Part model, mm, in its own coordinate system. A direction names the side the tool comes from. Round coordinates to 2 decimals unless told otherwise and drop trailing zeros. Order: outer loops, then holes, each group sorted by start corner. A loop starts at its lowest first (then second) coordinate and runs counter-clockwise, first axis right, second up. Notation, with made-up numbers: (23, -5) - (28, -5) arc R16 cw to (28, 18) - close; hole circle Ø8 at (44.5, 41.25). An arc over 180 degrees is marked (long way). Answer as a JSON object with one key per item and string values.
```python
from build123d import *

# Parameters (mm, degrees)
F1_DEPTH = 5
F3_DEPTH = 100
F4_SIZE  = 1


with BuildPart() as f1:
    # F0 (on Front) → F1 (new body)
    with BuildSketch(Plane.XZ):
        Polygon((66.3298651576, -50.2631962299), (66.3298651576, 49.7368037701), (-33.6701348424, 49.7368037701), (-33.6701348424, -50.2631962299), (-3.6701348424, -50.2631962299), (-3.6701348424, -20.2631962299), (16.3298651576, -20.2631962299), (36.3298651576, -20.2631962299), (36.3298651576, -50.2631962299), align=None)
    extrude(amount=F1_DEPTH)

    # F2 (on face) → F3 (cut)
    with BuildSketch(Plane(origin=(-33.6701348424, 0, 0), x_dir=(0, -1, 0), z_dir=(-1, 0, 0))):
        Polygon((2, -40.2631962299), (5, -40.2631962299), (5, -20.2631962299), (4, -20.2631962299), (4, -30.2631962299), (2, -30.2631962299), align=None)
    extrude(amount=-F3_DEPTH, mode=Mode.SUBTRACT)

    # F4
    f4_edges = [f1.edges().sort_by_distance(p)[0] for p in [
        (66.329865, 0, -0.263196),
        (16.329865, 0, 49.736804),
        (-33.670135, 0, -0.263196),
        (-18.670135, 0, -50.263196),
        (-3.670135, 0, -35.263196),
        (16.329865, 0, -20.263196),
        (36.329865, 0, -35.263196),
        (51.329865, 0, -50.263196),
        (66.329865, -5, -45.263196),
        (51.329865, -5, -50.263196),
        (36.329865, -5, -45.263196),
        (-3.670135, -5, -45.263196),
        (-18.670135, -5, -50.263196),
        (-33.670135, -5, -45.263196),
        (66.329865, -2.5, -50.263196),
        (36.329865, -2.5, -50.263196),
        (-3.670135, -2.5, -50.263196),
        (-33.670135, -2.5, -50.263196),
        (-33.670135, -2.5, 49.736804),
        (66.329865, -2.5, 49.736804),
        (-33.670135, -5, 14.736804),
        (16.329865, -5, 49.736804),
        (66.329865, -5, 14.736804),
    ]]
    chamfer(f4_edges, length=F4_SIZE)


solid = f1.part
```
Item 1: Cut at B-B (x = -8.5). Write the cut outline in (y, z), plus the area to 3 significant figures.
Taken from the geometry:
{"outline": "(-5, -49.26) - (-4, -50.26) - (-1, -50.26) - (0, -49.26) - (0, 48.74) - (-1, 49.74) - (-4, 49.74) - (-5, 48.74) - (-5, -20.26) - (-4, -20.26) - (-4, -30.26) - (-2, -30.26) - (-2, -40.26) - (-5, -40.26) - close", "area": "458 mm2"}
Item 2: Two-plate mould, pull along X, no slides. Class faces 4 (the flat face through (-33.67, -2, 0)), 5 (the flat face through (-19, -2, -35)), 6 (the flat face through (16, -3, -20.263)): pulls with the +X half, pulls with the -X half, needs draft (parallel to the pull), parting line crosses it, or undercut.
Taken from the geometry:
{"face 4": "pulls with the -X half", "face 5": "needs draft", "face 6": "undercut"}
Item 3: Probe L1, parallel to X at y = -2.7, z = -29; L2, parallel to Z at x = 38.5, y = -2.7; L3, parallel to Y at x = 59, z = -36. List the from-to ranges inside material, lowest first. Write a range as from..to.
Taken from the geometry:
{"L1": "-33.67..-3.67, 36.33..66.33", "L2": "-50.26..-40.26, -30.26..49.74", "L3": "-2..0"}
Item 4: Cut at C-C (x = 32.5). Write the cut outline in (y, z).
Taken from the geometry:
{"outline": "(-5, -20.26) - (-1, -20.26) - (0, -19.26) - (0, 48.74) - (-1, 49.74) - (-4, 49.74) - (-5, 48.74) - close"}
Item 5: Cut at A-A (z = -36.5). Write the cut outline in (x, y).
Taken from the geometry:
{"outline": "(-33.67, -2) - (-3.67, -2) - (-3.67, -1) - (-4.67, 0) - (-32.67, 0) - (-33.67, -1) - close; (36.33, -2) - (66.33, -2) - (66.33, -1) - (65.33, 0) - (37.33, 0) - (36.33, -1) - close"}
Item 6: Tool access for faces 1 (the flat face through (-19, -4, -25)), 2 (the flat face through (-19, -2, -50.263)), 3 (the flat face through (36.33, -1.8, -34.6)): list every direction of +Z, -Z, +X, -X, +Y, -Y with a clear straight run to the whole face (end or side of a thin tool).
Taken from the geometry:
{"face 1": "+X, -X, -Y", "face 2": "-Z, +X, -X, +Y, -Y", "face 3": "-Z, +Y, -Y"}
Item 7: Drop flat-ended pins along their axis: P1, Ø3, axis at x = 6.5, y = -4, coming from the -Z side; P2, Ø3, axis at x = -12, z = -27, coming from the -Y side. Give the stop position or say it passes through.
Taken from the geometry:
{"P1": "z = -20.26", "P2": "y = -4"}
